Part model, mm, in its own coordinate system. A direction names the side the tool comes from. Give positions to 0.01 mm unless a question says otherwise; leave off trailing zeros. Write each loop counter-clockwise with the first axis right and the second up, starting at its lowest first coordinate (ties: lowest second). Pieces come first, ordered by that corner, then holes. Notation, with made-up numbers: M 2.5,-17 L 43.5,-17 A19 cw 43.5,-1 Z; hole C 27,71.5 d4. An arc over 180 degrees is marked long. Use CSV: the item, a comma, the result in double quotes. Start each with the question number.
1. Band-saw the part on D-D, the plane z = -6.25. List the corners of the cut face in (x, y), then the cut area to 3 significant figures.
2. Band-saw the part on C-C, the plane y = 151.5. List the corners of the cut face in (x, z), then the cut area to 3 significant figures.
3. Drop flat-ended pins along their axis: pin 1 Ø0.9 at (x, y) = (-0.5, 116) entering from +Z; pin 2 Ø5 at (y, z) = (36, -8.5) entering from -X; pin 3 Ø3 at (x, y) = (-4, 40.5) entering from -Z (3 decimals). Give the stop position or say it passes through.
4. Band-saw the part on A-A, the plane x = 0. List the corners of the cut face in (y, z), then the cut area to 3 significant figures.
5. Band-saw the part on B-B, the plane z = 2.5. List the corners of the cut face in (x, y), then the cut area to 3 significant figures.
6. Drill centre lines: line 1 along Y through (x, z) = (0, 6); line 2 along Y through (x, z) = (1, 3.75); line 3 along X through (y, z) = (116.62, 2.5). Where is each one in solid material? Low to high. Write a range as from..to.
7. 3-axis set-ups, long thin cutter, end or side, ignore diameter. For faces 4 (the face through (0, 0, 0)), 5 (the face through (0, 53, 0)): which of +Z, -Z, +X, -X, +Y, -Y reach the whole face in a straight line?
8. Mould opens along X. For faces 1 (the face through (-0.325, 115.156, 5.671)), 2 (the face through (-1.5, 83.8, -11.4)), 3 (the face through (0, 170, 0)) say: pulls with the +X half, pulls with the -X half, needs draft (parallel to the pull), parting line crosses it, or undercut.
from build123d import *

# Parameters (mm, degrees)
SKETCH2_R           = 11.5
BOSS_EXTRUDE1_DEPTH = 170
CUT_EXTRUDE1_REACH  = 13.5
SKETCH3_R           = 1.5


with BuildPart() as part:
    # Sketch2 → Boss-Extrude1 (new body)
    with BuildSketch(Plane(origin=(0, 0, 0), x_dir=(1, 0, 0), z_dir=(0, 1, 0))):
        Circle(SKETCH2_R)
    extrude(amount=BOSS_EXTRUDE1_DEPTH)

    # Sketch3 → Cut-Extrude1 (cut, up to next)
    with BuildSketch(Plane.XY, mode=Mode.PRIVATE) as cut_extrude1_sk1:
        with Locations((0, 53.38)):
            Circle(SKETCH3_R)
    cut_extrude1_tool1 = extrude(cut_extrude1_sk1.sketch, amount=CUT_EXTRUDE1_REACH, mode=Mode.PRIVATE) & part.part
    add(cut_extrude1_tool1.solids().sort_by_distance((0, 53.38, 0))[0], mode=Mode.SUBTRACT)
    # Sketch3 → Cut-Extrude1 (cut, up to next)
    with BuildSketch(Plane.XY, mode=Mode.PRIVATE) as cut_extrude1_sk2:
        with Locations((0, 116.62)):
            Circle(SKETCH3_R)
    cut_extrude1_tool2 = extrude(cut_extrude1_sk2.sketch, amount=CUT_EXTRUDE1_REACH, mode=Mode.PRIVATE) & part.part
    add(cut_extrude1_tool2.solids().sort_by_distance((0, 116.62, 0))[0], mode=Mode.SUBTRACT)


solid = part.part
Output:
1,outline,"M -9.65,0 L 9.65,0 L 9.65,170 L -9.65,170 Z"
1,area,"3,280 mm²"
2,outline,"C 0,0 d23"
2,area,"415 mm²"
3,pin 1,"stops at z = 0"
3,pin 2,"stops at x = -9.81"
3,pin 3,"stops at z = -11.225"
4,outline,"M 0,-11.5 L 170,-11.5 L 170,11.5 L 118.12,11.5 L 118.12,0 L 115.12,0 L 115.12,11.5 L 54.88,11.5 L 54.88,0 L 51.88,0 L 51.88,11.5 L 0,11.5 Z"
4,area,"3,840 mm²"
5,outline,"M -11.22,0 L 11.22,0 L 11.22,170 L -11.22,170 Z; hole C 0,53.38 d3; hole C 0,116.62 d3"
5,area,"3,800 mm²"
6,line 1,"y = 0..51.88, 54.88..115.12, 118.12..170"
6,line 2,"y = 0..52.26, 54.5..115.5, 117.74..170"
6,line 3,"x = -11.22..-1.5, 1.5..11.22"
7,face 4,"+Z, -Z, +X, -X, -Y"
7,face 5,"+Z"
8,face 1,"undercut"
8,face 2,"parting line crosses it"
8,face 3,"needs draft"
